```python
from build123d import *

# Parameters (mm, degrees)
SKETCH1_W               = 110
SKETCH1_H               = 110
SKETCH1_R               = 1.55
SKETCH1_R_2             = 1.05
SKETCH1_R_3             = 1.5
BOSS_EXTRUDE2_DEPTH     = 3
SKETCH3_W               = 25
SKETCH3_H               = 25
CUT_EXTRUDE1_DEPTH      = 3
SKETCH4_R               = 5
BOSS_EXTRUDE3_DEPTH     = 3
SKETCH5_R               = 1.5
CUT_EXTRUDE3_DEPTH      = 4
SKETCH6_W               = 60
SKETCH6_H               = 1.5
CUT_EXTRUDE6_DEPTH      = 1
CUT_EXTRUDE6_DEPTH_BACK = 4


with BuildPart() as part:
    # Sketch1 → Boss-Extrude2 (new body)
    with BuildSketch(Plane(origin=(0, 0, 0), x_dir=(1, 0, 0), z_dir=(0, 1, 0))):
        Rectangle(SKETCH1_W, SKETCH1_H)
        with Locations((-48.6, 18.35)):
            Circle(SKETCH1_R, mode=Mode.SUBTRACT)
        with Locations((-11.9, 18.35)):
            Circle(SKETCH1_R, mode=Mode.SUBTRACT)
        with Locations((-11.9, -18.35)):
            Circle(SKETCH1_R, mode=Mode.SUBTRACT)
        with Locations((-48.6, -18.35)):
            Circle(SKETCH1_R, mode=Mode.SUBTRACT)
        with Locations((48.6, -18.35)):
            Circle(SKETCH1_R, mode=Mode.SUBTRACT)
        with Locations((11.9, -18.35)):
            Circle(SKETCH1_R, mode=Mode.SUBTRACT)
        with Locations((11.9, 18.35)):
            Circle(SKETCH1_R, mode=Mode.SUBTRACT)
        with Locations((48.6, 18.35)):
            Circle(SKETCH1_R, mode=Mode.SUBTRACT)
        with Locations((-24.5, 47.2)):
            Circle(SKETCH1_R_2, mode=Mode.SUBTRACT)
        with Locations((-24.5, 35.8)):
            Circle(SKETCH1_R_2, mode=Mode.SUBTRACT)
        with Locations((22.5, 47.2)):
            Circle(SKETCH1_R_2, mode=Mode.SUBTRACT)
        with Locations((22.5, 35.8)):
            Circle(SKETCH1_R_2, mode=Mode.SUBTRACT)
        with Locations((-15, -33.5)):
            Circle(SKETCH1_R_3, mode=Mode.SUBTRACT)
        with Locations((15, -49.5)):
            Circle(SKETCH1_R_3, mode=Mode.SUBTRACT)
    extrude(amount=BOSS_EXTRUDE2_DEPTH)

    # Sketch3 → Cut-Extrude1 (cut)
    with BuildSketch(Plane(origin=(0, 3, 0), x_dir=(1, 0, 0), z_dir=(0, 1, 0))):
        with Locations((42.5, 42.5)):
            Rectangle(SKETCH3_W, SKETCH3_H)
        with Locations((-42.5, 42.5)):
            Rectangle(SKETCH3_W, SKETCH3_H)
        with Locations((42.5, -42.5)):
            Rectangle(SKETCH3_W, SKETCH3_H)
        with Locations((-42.5, -42.5)):
            Rectangle(SKETCH3_W, SKETCH3_H)
    extrude(amount=-CUT_EXTRUDE1_DEPTH, mode=Mode.SUBTRACT)

    # Sketch4 → Boss-Extrude3 (add)
    with BuildSketch(Plane(origin=(0, 3, 0), x_dir=(1, 0, 0), z_dir=(0, 1, 0))):
        with Locations((50, 30)):
            Circle(SKETCH4_R)
        with Locations((-50, 30)):
            Circle(SKETCH4_R)
        with Locations((50, -30)):
            Circle(SKETCH4_R)
        with Locations((-50, -30)):
            Circle(SKETCH4_R)
        with Locations((-25, 55)):
            Circle(SKETCH4_R)
        with Locations((25, 55)):
            Circle(SKETCH4_R)
        with Locations((25, -55)):
            Circle(SKETCH4_R)
        with Locations((-25, -55)):
            Circle(SKETCH4_R)
    extrude(amount=-BOSS_EXTRUDE3_DEPTH)

    # Sketch5 → Cut-Extrude3 (cut, through all)
    with BuildSketch(Plane(origin=(0, 3, 0), x_dir=(1, 0, 0), z_dir=(0, 1, 0))):
        with Locations((50, 30)):
            Circle(SKETCH5_R)
        with Locations((50, -30)):
            Circle(SKETCH5_R)
        with Locations((-50, -30)):
            Circle(SKETCH5_R)
        with Locations((-50, 30)):
            Circle(SKETCH5_R)
        with Locations((-25, 55)):
            Circle(SKETCH5_R)
        with Locations((25, 55)):
            Circle(SKETCH5_R)
        with Locations((25, -55)):
            Circle(SKETCH5_R)
        with Locations((-25, -55)):
            Circle(SKETCH5_R)
    extrude(amount=-CUT_EXTRUDE3_DEPTH, mode=Mode.SUBTRACT)

    # Sketch6 → Cut-Extrude6 (cut, two sides)
    with BuildSketch(Plane(origin=(0, 3, 0), x_dir=(1, 0, 0), z_dir=(0, 1, 0))) as cut_extrude6_sk:
        with Locations((0, 59.25)):
            Rectangle(SKETCH6_W, SKETCH6_H)
        with Locations((0, -59.25)):
            Rectangle(SKETCH6_W, SKETCH6_H)
    extrude(amount=CUT_EXTRUDE6_DEPTH, mode=Mode.SUBTRACT)
    extrude(cut_extrude6_sk.sketch, amount=-CUT_EXTRUDE6_DEPTH_BACK, mode=Mode.SUBTRACT)


solid = part.part
```
Design review of the part built by this model. Coordinates are the model's own, in mm. A direction names the side the tool comes from. Round coordinates to 2 decimals unless told otherwise and drop trailing zeros. Write each loop counter-clockwise with the first axis right and the second up, starting at its lowest first coordinate (ties: lowest second). Pieces come first, ordered by that corner, then holes.
Item 1: The part is to be moulded in two halves that separate along Z. For faces 1 (the flat face through (55, 1, 0)), 2 (the cylindrical face through (29.639, 1.521, -56.865)), 3 (the cylindrical face through (-51.11, 1.52, 28.99)), say which applies: +Z half, -Z half, draft (parallel to the pull), parting line (faces both ways), or undercut.
Item 2: For faces 4 (the cylindrical face through (-51.5, 1.52, -30.07)), 5 (the cylindrical face through (20.361, 1.521, 56.865)), 6 (the cylindrical face through (20.381, 1.521, -56.915)), list the 3-axis set-ups (+Z, -Z, +X, -X, +Y, -Y) from which the entire face can be reached by the end or side of a thin tool; tool diameter is ignored.
Item 3: For probe 1 along Z at (x, y) = (25, 1.3); probe 2 along X at (y, z) = (1.55, 18.35); probe 3 along Z at (x, y) = (12, 1.5), list the stretches that pass through material, from the lowest coordinate up.
Item 4: We need section B-B on x = 11.9. Write out the cut boundary in (y, z), and give its area (3 significant figures).
Item 5: We need section A-A on x = 25. Write out the cut boundary in (y, z).
Item 6: Clearance check with flat-ended pins moving along their axes: pin 1 Ø0.9 at (x, y) = (-36.5, 2) entering from -Z; pin 2 Ø2.5 at (x, z) = (22.5, -47.2) entering from +Y; pin 3 Ø1 at (x, y) = (20, 1) entering from +Z; pin 4 Ø0.9 at (y, z) = (1.5, 37.5) entering from +X. State where each tip first meets the part, or that it passes through.
Item 7: We need section D-D on x = -34. Write out the cut boundary in (y, z), and give its area (3 significant figures).
Item 8: We need section C-C on y = 1.35. State how many separate pieces and enclosed holes the cut face has, and give its area (3 significant figures).
Returned:
1. face 1: draft
1. face 2: -Z half
1. face 3: undercut
2. face 4: +Y, -Y
2. face 5: +Z, +Y, -Y
2. face 6: -Z, +Y, -Y
3. probe 1: z = -58.5 to -56.5, -53.5 to 53.5, 56.5 to 58.5
3. probe 2: x = -55 to -50.15, -47.05 to -13.45, -10.35 to 10.35, 13.45 to 47.05, 50.15 to 55
3. probe 3: z = -55 to -19.9, -16.8 to 16.8, 19.9 to 55
4. outline: (0, -55) - (3, -55) - (3, -19.9) - (0, -19.9) - close; (0, -16.8) - (3, -16.8) - (3, 16.8) - (0, 16.8) - close; (0, 19.9) - (3, 19.9) - (3, 55) - (0, 55) - close
4. area: 311 mm2
5. outline: (0, -58.5) - (3, -58.5) - (3, -56.5) - (0, -56.5) - close; (0, -53.5) - (3, -53.5) - (3, 53.5) - (0, 53.5) - close; (0, 56.5) - (3, 56.5) - (3, 58.5) - (0, 58.5) - close
6. pin 1: stops at z = -30
6. pin 2: stops at y = 3
6. pin 3: stops at z = 57.18
6. pin 4: stops at x = 30
7. outline: (0, -30) - (3, -30) - (3, 30) - (0, 30) - close
7. area: 180 mm2
8. separate pieces: 1
8. enclosed holes: 22
8. area: 9,740 mm2
